```python
from build123d import *

# Parameters (mm, degrees)
F0_W     = 95.25
F0_H     = 76.2
F1_DEPTH = 38.1
F1_TAPER = 3
F2_R     = 5.08
F4_D     = 31.75
F4_DEPTH = 12.7
F4_TIP   = 9.5386623271


with BuildPart() as f1:
    # F0 (on Front) → F1 (new body, symmetric)
    with BuildSketch(Plane.XZ):
        with Locations((-1.951872288, -1.5614978304)):
            Rectangle(F0_W, F0_H)
    extrude(amount=F1_DEPTH, both=True, taper=F1_TAPER)

    # F2
    f2_edges = [f1.edges().sort_by_distance(p)[0] for p in [
        (43.676391, -38.1, -1.561498),
        (-1.951872, -38.1, 34.541766),
        (-47.580136, -38.1, -1.561498),
        (-1.951872, -38.1, -37.664761),
        (43.676391, 38.1, -1.561498),
        (-1.951872, 38.1, 34.541766),
        (-47.580136, 38.1, -1.561498),
        (-1.951872, 38.1, -37.664761),
        (44.67476, -19.05, 35.540134),
        (44.67476, -19.05, -38.66313),
        (44.67476, 19.05, 35.540134),
        (44.67476, 19.05, -38.66313),
        (-48.578504, -19.05, 35.540134),
        (-48.578504, -19.05, -38.66313),
        (-48.578504, 19.05, 35.540134),
        (-48.578504, 19.05, -38.66313),
    ]]
    fillet(f2_edges, radius=F2_R)

    # F4
    with Locations(Plane(origin=(0, 38.1, 0), x_dir=(-1, 0, 0), z_dir=(0, 1, 0))):
        with Locations((0, 0)):
            Hole(F4_D / 2, depth=F4_DEPTH)
            with Locations((0, 0, -(F4_DEPTH + F4_TIP / 2))):  # 118° drill point
                Cone(0, F4_D / 2, F4_TIP, mode=Mode.SUBTRACT)


solid = f1.part
```
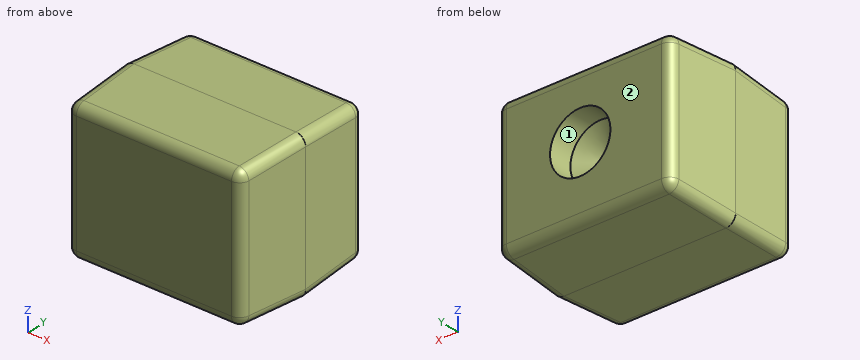
Read the model definition and answer for the solid it produces. Units are mm, in the model's axes. Face numbers are marked on the shaded views. Give positions to 0.01 mm unless a question says otherwise; leave off trailing zeros. Write item = value, one per line.
1. Straight lines are drawn through the part: line 1 along Z through (x, y) = (0, 33) (3 decimals); line 2 along X through (y, z) = (34.5, 0) (3 decimals); line 3 along X through (y, z) = (31, 0) (3 decimals). For each, find the intervals that lie inside material, in ascending order.
Numbers:
line_1 = -37.932 to -15.875, 15.875 to 34.809
line_2 = -47.619 to -15.875, 15.875 to 43.715
line_3 = -47.952 to -15.875, 15.875 to 44.048
2. Given pin 1 (10 mm diameter, centred on y = -19.5, z = -23, fed in from -X); pin 2 (5 mm diameter, centred on x = 33.5, y = 9, fed in from -Z); pin 3 (2 mm diameter, centred on y = -1, z = -7, fed in from +X); pin 4 (4 mm diameter, centred on x = -31.5, y = -9.5, fed in from +Z), each flat-ended and moving along its own axis, determine where each tip first touches the part or whether it passes through.
Numbers:
pin_1 = -48.82
pin_2 = -39.32
pin_3 = 45.67
pin_4 = 36.15
3. The mould has two halves that part along X. Classify the marked faces 1 and 2: +X half, -X half, draft (parallel to the pull), parting line (faces both ways), or undercut.
Numbers:
face_1 = undercut
face_2 = draft
